Print and shaded views of the part. All mm, measured from the part's lowest x, y and z. A direction names the side the tool comes from. Coordinates: 2 decimals unless noted, no trailing zeros. Loops run counter-clockwise (first coordinate to the right, second up) from the corner with the lowest first, then second, coordinate; pieces in that order, holes last. Notation, with made-up numbers: (28.25, -16) -> (78.25, -16) arc R30 cw to (78.25, 9) -> close; hole circle Ø7 at (49.5, -16.5). An arc over 180 degrees is marked (long way). One line per item, written item: value. Start each with the question number.
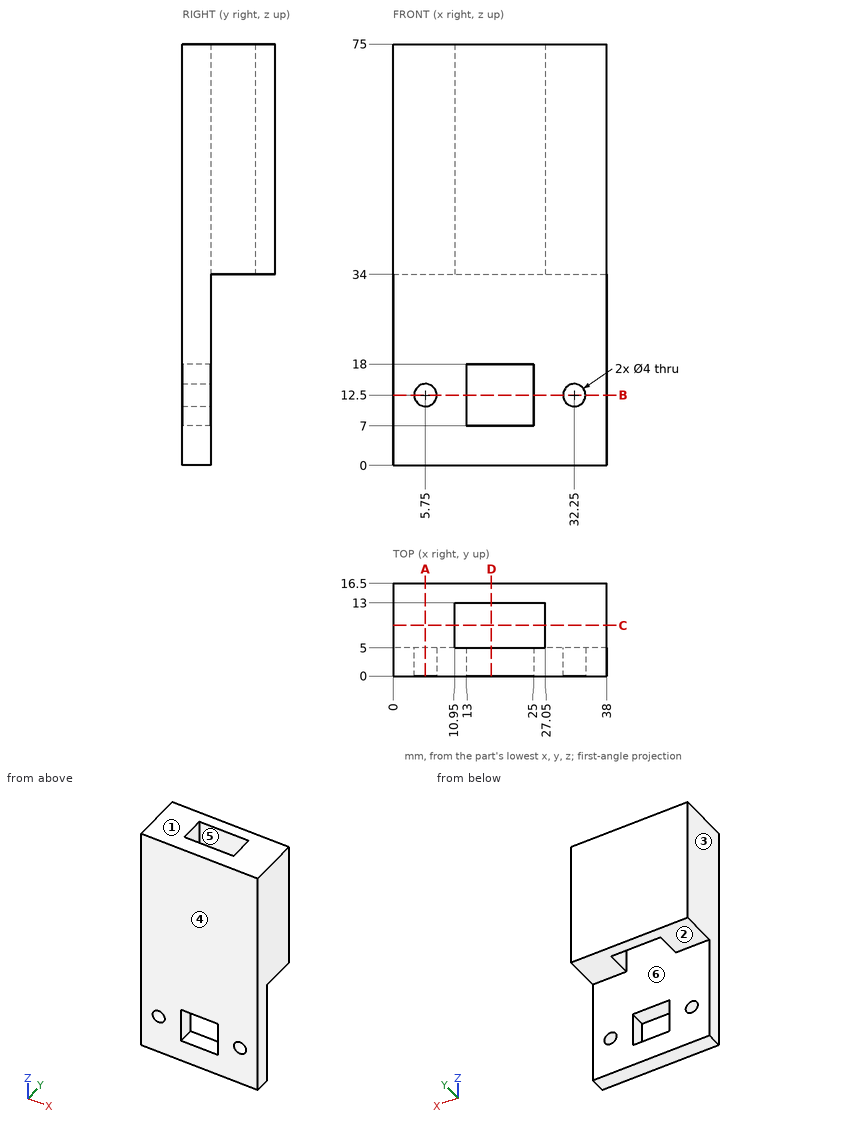
1) Probe line 1 (Z direction, x = 24, y = 3.25); line 2 (Y direction, x = 24, z = 50.5); line 3 (Z direction, x = 5.75, y = 2.45). List the from-to ranges inside material, lowest first. Write a range as from..to.
2) Tool access for the marked faces 1 and 2: list every direction of +Z, -Z, +X, -X, +Y, -Y with a clear straight run to the whole face (end or side of a thin tool).
3) Slice it at D-D (x = 17.5). Give the cut face in (y, z).
4) Slice it at A-A (x = 5.75). Give the cut face in (y, z).
5) Slice it at C-C (y = 9). Give the cut face in (x, z).
6) Slice it at B-B (z = 12.5). Give the cut face in (x, y).
7) Pin check, flat tips, straight feed: pin 1 Ø2 at (y, z) = (3.5, 64.5) entering from -X; pin 2 Ø6 at (x, y) = (15, 14) entering from -Z. Stop position of each tip, or through.
8) Pull direction Y, two halves, no side cores. Call the marked faces 3, 4, 5 and 6: +Y half, -Y half, draft (parallel to the pull), parting line (faces both ways), or undercut.
Check sheet entries:
1. line 1: z = 0..7, 18..75
1. line 2: y = 0..5, 13..16.5
1. line 3: z = 0..10.5, 14.5..75
2. face 1: +Z, +X, -X, +Y, -Y
2. face 2: -Z, +X, -X, +Y
3. outline: (0, 0) -> (5, 0) -> (5, 7) -> (0, 7) -> close; (0, 18) -> (5, 18) -> (5, 75) -> (0, 75) -> close; (13, 34) -> (16.5, 34) -> (16.5, 75) -> (13, 75) -> close
4. outline: (0, 0) -> (5, 0) -> (5, 10.5) -> (0, 10.5) -> close; (0, 14.5) -> (5, 14.5) -> (5, 34) -> (16.5, 34) -> (16.5, 75) -> (0, 75) -> close
5. outline: (0, 34) -> (10.95, 34) -> (10.95, 75) -> (0, 75) -> close; (27.05, 34) -> (38, 34) -> (38, 75) -> (27.05, 75) -> close
6. outline: (0, 0) -> (3.75, 0) -> (3.75, 5) -> (0, 5) -> close; (7.75, 0) -> (13, 0) -> (13, 5) -> (7.75, 5) -> close; (25, 0) -> (30.25, 0) -> (30.25, 5) -> (25, 5) -> close; (34.25, 0) -> (38, 0) -> (38, 5) -> (34.25, 5) -> close
7. pin 1: stops at x = 0
7. pin 2: stops at z = 34
8. face 3: draft
8. face 4: -Y half
8. face 5: undercut
8. face 6: undercut
